The model under review builds one solid part; all positions refer to its coordinate system, in mm. Round coordinates to 2 decimals unless told otherwise and drop trailing zeros. Order: outer loops, then holes, each group sorted by start corner. A loop starts at its lowest first (then second) coordinate and runs counter-clockwise, first axis right, second up. Notation, with made-up numbers: M 56.5,89.5 L 110.5,89.5 A24 cw 110.5,126.5 Z; hole C 19.25,33.25 d4. An arc over 180 degrees is marked long. Answer as a JSON object with one key per item and string values. Group by question number.
1. Add section B-B on y = -31.5. State the section outline as (x, z) points.
2. To check wall thickness, follow probe 1 along Y at (x, z) = (-1.5, 0.3); probe 2 along Y at (x, z) = (-19, 2.5); probe 3 along X at (y, z) = (-33, 1.4). State the ranges of each line that lie inside material, in increasing order. Write a range as [from, to].
3. Add section A-A on x = -10. State the section outline as (y, z) points.
4. Clearance check with flat-ended pins moving along their axes: P1, Ø1.4, axis at y = -34, z = 1.5, coming from the +X side; P2, Ø1.5, axis at x = -17, z = 2, coming from the -Y side; P3, Ø0.8, axis at y = -32.5, z = 1, coming from the +X side. State where each tip first meets the part, or that it passes through.
```python
from build123d import *

# Parameters (mm, degrees)
SALIENTE_EXTRUIR1_DEPTH = 3
REDONDEO1_R             = 1
REDONDEO2_R             = 0.25


with BuildPart() as part:
    # Croquis1 → Saliente-Extruir1 (new body)
    with BuildSketch(Plane.XY):
        with BuildLine():
            Line((-7, 27.5), (-7, 34))
            ThreePointArc((-7, 34), (-6.267766953, 35.767766953), (-4.5, 36.5))
            Line((-4.5, 36.5), (3, 36.5))
            Line((3, 36.5), (3, 33.5))
            Line((3, 33.5), (-2, 33.5))
            Line((-2, 33.5), (-2, 30.5))
            Line((-2, 30.5), (3, 30.5))
            Line((3, 30.5), (3, 27.5))
            Line((3, 27.5), (25, 27.5))
            Line((25, 27.5), (25, -27.5))
            Line((25, -27.5), (3, -27.5))
            Line((3, -27.5), (3, -30.5))
            Line((3, -30.5), (-2, -30.5))
            Line((-2, -30.5), (-2, -33.5))
            Line((-2, -33.5), (3, -33.5))
            Line((3, -33.5), (3, -36.5))
            Line((3, -36.5), (-4.5, -36.5))
            ThreePointArc((-4.5, -36.5), (-6.267766953, -35.767766953), (-7, -34))
            Line((-7, -34), (-7, -27.5))
            Line((-7, -27.5), (-25, -27.5))
            Line((-25, -27.5), (-25, 27.5))
            Line((-25, 27.5), (-7, 27.5))
        make_face()
    extrude(amount=SALIENTE_EXTRUIR1_DEPTH)

    # Redondeo1
    redondeo1_edges = [part.edges().sort_by_distance(p)[0] for p in [
        (-25, 27.5, 1.5),
        (-25, -27.5, 1.5),
        (-7, -27.5, 1.5),
        (3, -36.5, 1.5),
        (3, -27.5, 1.5),
        (25, -27.5, 1.5),
        (25, 27.5, 1.5),
        (3, 27.5, 1.5),
        (3, 36.5, 1.5),
        (-7, 27.5, 1.5),
    ]]
    fillet(redondeo1_edges, radius=REDONDEO1_R)

    # Redondeo2
    redondeo2_edges = [part.edges().sort_by_distance(p)[0] for p in [
        (3, -33.5, 1.5),
        (-2, -33.5, 1.5),
        (-2, -30.5, 1.5),
        (3, -30.5, 1.5),
        (3, 30.5, 1.5),
        (-2, 30.5, 1.5),
        (-2, 33.5, 1.5),
        (3, 33.5, 1.5),
    ]]
    fillet(redondeo2_edges, radius=REDONDEO2_R)


solid = part.part
```
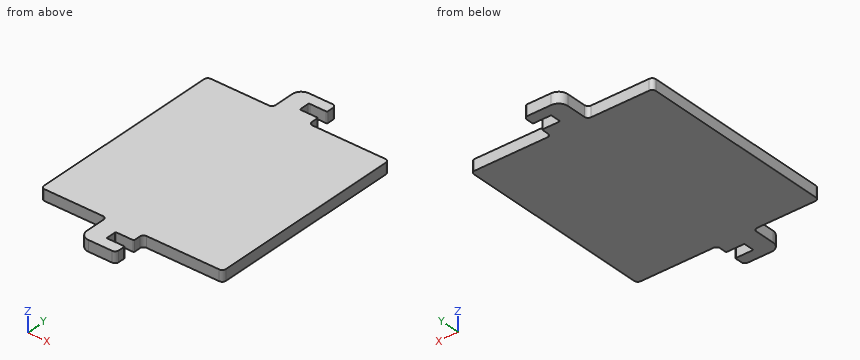
Recorded:
{
 "1": {"outline": "M -7,0 L -2,0 L -2,3 L -7,3 Z"},
 "2": {"probe 1": "y = [-36.5, -33.5], [-30.5, 30.5], [33.5, 36.5]", "probe 2": "y = [-27.5, 27.5]", "probe 3": "x = [-7, -2]"},
 "3": {"outline": "M -27.5,0 L 27.5,0 L 27.5,3 L -27.5,3 Z"},
 "4": {"P1": "stops at x = 3", "P2": "stops at y = -27.5", "P3": "stops at x = -2"}
}
